Geometry check sheet. Reference: the model listing, model coordinates, mm. A direction names the side the tool comes from. Give positions to 0.01 mm unless a question says otherwise; leave off trailing zeros. Write each loop counter-clockwise with the first axis right and the second up, starting at its lowest first coordinate (ties: lowest second). Pieces come first, ordered by that corner, then holes. Notation, with made-up numbers: (78, 89) - (118, 89) arc R25 cw to (118, 108) - close; hole circle Ø4 at (-26, 30). An arc over 180 degrees is marked (long way). One line per question, with ' | ' between items. Start each with the question number.
Q1. Thickness scan on L1, parallel to Z at x = -14.5, y = 6; L2, parallel to X at y = 10, z = 81.5; L3, parallel to X at y = 3, z = 58.5. Record the ranges inside material, lowest first. Write a range as [from, to].
Q2. Gauge pin test, flat ends, axial feed: P1, Ø3, axis at x = -88, z = 43, coming from the -Y side (3 decimals); P2, Ø6, axis at y = 6, z = 10.84, coming from the -X side; P3, Ø4, axis at x = -90, y = -19.5, coming from the -Z side; P4, Ø8, axis at x = -53.5, z = 48.5, coming from the -Y side. Record the tip position at first contact, or that the pin passes through.
Q3. Set-up check for faces 4 (the face through (-42.76, -0.77, 50.55)), 5 (the face through (-91.39, -14.84, 50.45)), 6 (the face through (-61, -9, 75)), 7 (the face through (-20, 6, 15)): record each of +Z, -Z, +X, -X, +Y, -Y from which the full face is reachable in a straight line by a thin tool's end or side.
Q4. Section check A-A on y = 7. Record the boundary of the cut face in (x, z).
Q5. Section check B-B on x = -6.5. Record the boundary of the cut face in (y, z), and give its area (3 significant figures).
Q6. Section check C-C on z = 77. Record the boundary of the cut face in (x, y).
Q7. Release check for a two-part mould opening along X. For faces 1 (the face through (-45.36, 4.59, 49.65)), 2 (the face through (-88.936, -21.395, 50.451)), 3 (the face through (-68, -10, 63)) record: +X half, -X half, draft (parallel to the pull), parting line (faces both ways), or undercut.
```python
from build123d import *

# Parameters (mm, degrees)
F1_DEPTH  = 100
F3_W      = 46
F3_H      = 26
F4_DEPTH  = 25
F7_W      = 98.6057445407
F7_H      = 75.1156285405
F8_DEPTH  = 30
F10_W     = 97.911
F10_H     = 83.95
F11_DEPTH = 30
F15_R     = 2.5
F16_DEPTH = 30
F13_R     = 2.5
F17_DEPTH = 30
F19_W     = 7
F19_H     = 7
F20_DEPTH = 8
F22_W     = 7
F22_H     = 7
F23_DEPTH = 8


with BuildPart() as f1:
    # F0 (on Top) → F1 (new body)
    with BuildSketch(Plane.XY):
        Polygon((-25, 0), (0, 0), (0, 12), (-25, 12), (-100.1754096629, -15.3616114661), (-96.071167943, -26.6379229155), align=None)
    extrude(amount=F1_DEPTH)

    # F3 (on offset) → F4 (cut)
    with BuildSketch(Plane(origin=(-3.0794008865, 8.2159790861, 0), x_dir=(0.9363887892, 0.3509644362, 0), z_dir=(0.3509644362, -0.9363887892, 0))):
        with Locations((-66.3089282241, 50)):
            Rectangle(F3_W, F3_H)
    extrude(amount=-F4_DEPTH, mode=Mode.SUBTRACT)

    # F7 (on offset) → F8 (cut)
    with BuildSketch(Plane.XY.offset(105)):
        with Locations((-70.1127834618, -4.4539272785)):
            Rectangle(F7_W, F7_H)
    extrude(amount=-F8_DEPTH, mode=Mode.SUBTRACT)

    # F10 (on offset) → F11 (cut)
    with BuildSketch(Plane(origin=(0, 0, -5), x_dir=(1, 0, 0), z_dir=(0, 0, -1))):
        with Locations((-68.9555, -1.8251938164)):
            Rectangle(F10_W, F10_H)
    extrude(amount=-F11_DEPTH, mode=Mode.SUBTRACT)

    # F15 (on offset) → F16 (cut)
    with BuildSketch(Plane(origin=(-25, 0, 0), x_dir=(0, -1, 0), z_dir=(-1, 0, 0))):
        with Locations((-6, 10.8403703198)):
            Circle(F15_R)
    extrude(amount=-F16_DEPTH, mode=Mode.SUBTRACT)

    # F13 (on offset) → F17 (cut)
    with BuildSketch(Plane(origin=(-25.8099111915, 0, 0), x_dir=(0, -1, 0), z_dir=(-1, 0, 0))):
        with Locations((-6, 89.705966413)):
            Circle(F13_R)
    extrude(amount=-F17_DEPTH, mode=Mode.SUBTRACT)

    # F19 (on offset) → F20 (cut)
    with BuildSketch(Plane(origin=(-45.2359388073, -16.9547157565, 0), x_dir=(0.3509644362, -0.9363887892, 0), z_dir=(-0.9363887892, -0.3509644362, 0))):
        with Locations((-14.240679825, 50.5)):
            Rectangle(F19_W, F19_H)
    extrude(amount=-F20_DEPTH, mode=Mode.SUBTRACT)

    # F22 (on offset) → F23 (cut)
    with BuildSketch(Plane(origin=(-78.9459352184, -29.5894354589, 0), x_dir=(-0.3509644362, 0.9363887892, 0), z_dir=(0.9363887892, 0.3509644362, 0))):
        with Locations((14.6793034593, 50.5)):
            Rectangle(F22_W, F22_H)
    extrude(amount=-F23_DEPTH, mode=Mode.SUBTRACT)


solid = f1.part
```
Working result:
1) L1: z = [0, 8.34], [13.34, 87.21], [92.21, 100] | L2: x = [-20.81, 0] | L3: x = [-47.38, 0]
2) P1: stops at y = -24.175 | P2: stops at x = -20 | P3: stops at z = 25 | P4: passes through
3) face 4: none | face 5: +X | face 6: +Z, -X, +Y, -Y | face 7: -Z, -X, +Y, -Y
4) outline: (-38.74, 25) - (-20, 25) - (-20, 13.13) - (0, 13.13) - (0, 87.41) - (-20.81, 87.41) - (-20.81, 75) - (-38.74, 75) - close; (-20.81, 92) - (0, 92) - (0, 100) - (-20.81, 100) - close; (-20, 0) - (0, 0) - (0, 8.55) - (-20, 8.55) - close
5) outline: (0, 0) - (12, 0) - (12, 100) - (0, 100) - close; hole circle Ø5 at (6, 10.84); hole circle Ø5 at (6, 89.71) | area: 1,160 mm2
6) outline: (-20.81, 0) - (0, 0) - (0, 12) - (-20.81, 12) - close
7) face 1: -X half | face 2: undercut | face 3: draft
